Input: part model. Units: mm. Frame: model coordinates. A direction names the side the tool comes from. Give positions to 0.01 mm unless a question says otherwise; leave off trailing zeros. Order: outer loops, then holes, each group sorted by start corner. A loop starts at its lowest first (then second) coordinate and runs counter-clockwise, first axis right, second up. Notation, with made-up numbers: (0.5, 66.25) -> (38.5, 66.25) arc R35 cw to (38.5, 103.25) -> close; hole circle Ø6 at (89.25, 17). An arc over 180 degrees is marked (long way). Use a Markdown table: item, result. Add a question column.
from build123d import *

# Parameters (mm, degrees)
SKETCH1_W           = 115
SKETCH1_H           = 30
BOSS_EXTRUDE1_DEPTH = 10.5
CUT_EXTRUDE1_START  = 3
SKETCH2_R           = 11.1
CUT_EXTRUDE1_DEPTH  = 10.5
SKETCH3_R           = 6
CUT_EXTRUDE4_DEPTH  = 10.5
BOSS_EXTRUDE2_DEPTH = 10.5
SKETCH6_R           = 2.25
CUT_EXTRUDE5_DEPTH  = 10.5
SKETCH7_R           = 3
CUT_EXTRUDE6_DEPTH  = 7.5
CUT_EXTRUDE7_DEPTH  = 28.5
FILLET1_R           = 6
FILLET2_RADIUS      = 15
FILLET2_LENGTH      = 10.5


with BuildPart() as part:
    # Sketch1 → Boss-Extrude1 (new body)
    with BuildSketch(Plane(origin=(0, 0, 0), x_dir=(1, 0, 0), z_dir=(0, 1, 0))):
        Rectangle(SKETCH1_W, SKETCH1_H)
    extrude(amount=BOSS_EXTRUDE1_DEPTH)

    # Sketch2 → Cut-Extrude1 (cut)
    with BuildSketch(Plane(origin=(0, 0, 0), x_dir=(1, 0, 0), z_dir=(0, 1, 0)).offset(CUT_EXTRUDE1_START)):
        with Locations(Location((42.5, 0, 0), (0, 0, 90))):
            Circle(SKETCH2_R)
    extrude(amount=CUT_EXTRUDE1_DEPTH, mode=Mode.SUBTRACT)

    # Sketch3 → Cut-Extrude4 (cut)
    with BuildSketch(Plane(origin=(0, 0, 0), x_dir=(1, 0, 0), z_dir=(0, 1, 0))):
        with Locations(Location((42.5, 0, 0), (0, 0, 90))):
            Circle(SKETCH3_R)
    extrude(amount=CUT_EXTRUDE4_DEPTH, mode=Mode.SUBTRACT)

    # Sketch5 → Boss-Extrude2 (add)
    with BuildSketch(Plane(origin=(0, 0, 0), x_dir=(1, 0, 0), z_dir=(0, 1, 0))):
        Polygon((-57.5, 15), (-57.5, 25), (-37.5, 25), (-37.5, -25), (-57.5, -25), (-57.5, -15), align=None)
    extrude(amount=BOSS_EXTRUDE2_DEPTH)

    # Sketch6 → Cut-Extrude5 (cut)
    with BuildSketch(Plane(origin=(0, 10.5, 0), x_dir=(1, 0, 0), z_dir=(0, 1, 0))):
        with Locations(Location((-47.5, -15, 0), (0, 0, 270))):
            Circle(SKETCH6_R)
        with Locations(Location((-47.5, 15, 0), (0, 0, 270))):
            Circle(SKETCH6_R)
    extrude(amount=-CUT_EXTRUDE5_DEPTH, mode=Mode.SUBTRACT)

    # Sketch7 → Cut-Extrude6 (cut)
    with BuildSketch(Plane(origin=(0, 10.5, 0), x_dir=(1, 0, 0), z_dir=(0, 1, 0))):
        with Locations(Location((-47.5, 15, 0), (0, 0, 270))):
            Circle(SKETCH7_R)
        with Locations(Location((-47.5, -15, 0), (0, 0, 270))):
            Circle(SKETCH7_R)
    extrude(amount=-CUT_EXTRUDE6_DEPTH, mode=Mode.SUBTRACT)

    # Sketch8 → Cut-Extrude7 (cut)
    with BuildSketch(Plane(origin=(0, 10.5, 0), x_dir=(1, 0, 0), z_dir=(0, 1, 0))):
        Polygon((-37.5, 15), (-27.5, 7.5), (17.022877386, 7.5), (27.5, 15), align=None)
        Polygon((-37.5, -15), (27.5, -15), (17.022877386, -7.5), (-27.5, -7.5), align=None)
    extrude(amount=-CUT_EXTRUDE7_DEPTH, mode=Mode.SUBTRACT)

    # Fillet1
    fillet1_edges = [part.edges().sort_by_distance(p)[0] for p in [
        (-37.5, 5.25, -15),
        (-37.5, 5.25, 15),
        (-37.5, 5.25, 25),
        (-37.5, 5.25, -25),
        (27.5, 5.25, -15),
        (17.022877386, 5.25, -7.5),
        (-27.5, 5.25, -7.5),
        (-27.5, 5.25, 7.5),
        (17.022877386, 5.25, 7.5),
        (27.5, 5.25, 15),
    ]]
    fillet(fillet1_edges, radius=FILLET1_R)

    # Fillet2: full round fillet: the end face becomes a half cylinder, R = half its width
    fillet2_face = Plane((57.5, 5.25, 0), x_dir=(0, -1, 0), z_dir=(1, 0, 0))  # on the end face: x along it, z out of the body
    fillet2_slab = fillet2_face.offset(-FILLET2_RADIUS / 2) * Box(FILLET2_LENGTH, 2 * FILLET2_RADIUS, FILLET2_RADIUS, mode=Mode.PRIVATE)  # the body's end, R deep
    fillet2_round = Plane((42.5, 5.25, 0), x_dir=(1, 0, 0), z_dir=(0, -1, 0)) * Cylinder(FILLET2_RADIUS, FILLET2_LENGTH, mode=Mode.PRIVATE)  # its axis R under the face
    add(fillet2_slab - fillet2_round, mode=Mode.SUBTRACT)


solid = part.part
Q1. Ray query, line 1 (Z direction, x = 42.5, y = 1); line 2 (X direction, y = 6.25, z = 0); line 3 (Z direction, x = -26, y = 6.75). Return the intervals inside material, ascending.
Q2. Access query for faces 1 (the flat face through (36, 5, 15)), 2 (the cylindrical face through (31.494, 6.698, 1.445)), 3 (the flat face through (-5, 5, -7.5)), 4 (the flat face through (-5, 5, 7.5)). Directions: +Z, -Z, +X, -X, +Y, -Y. A direction counts if a zero-diameter tool reaches every point of the face in a straight line with its end or side. Return the directions, or none.
Q3. Section query A-A (z = 0). Return loops of the section in (x, y).
Q4. Draft query along Z for faces 5 (the flat face through (22.313, 5.324, 11.287)), 6 (the flat face through (22.21, 5.324, -11.213)), 7 (the cylindrical face through (48.357, 1.479, 1.301)). Return one class per face: +Z half, -Z half, draft (parallel to the pull), parting line (faces both ways), or undercut.
Q5. Section query C-C (x = 46). Return loops of the section in (y, z).
Q6. Section query B-B (y = 4.5). Return loops of the section in (x, z), plus the area to 3 significant figures.
Q7. Section query D-D (x = -22). Return loops of the section in (y, z), plus the area to 4 significant figures.
Q8. First-contact query: pin 1 (5 mm diameter, centred on x = -6, y = 6.5, fed in from -Z); pin 2 (3 mm diameter, centred on x = 31, y = 7.5, fed in from +Z); pin 3 (1.8 mm diameter, centred on x = -49, z = 16, fed in from +Y). Flat tips, straight axial feed; report the tip coordinate or a pass-through.
Solution:
| question | item | result |
|---|---|---|
| 1 | line 1 | z = -15 to -6, 6 to 15 |
| 1 | line 2 | x = -57.5 to 31.4, 53.6 to 57.5 |
| 1 | line 3 | z = -7.52 to 7.52 |
| 2 | face 1 | +Z, +X, +Y, -Y |
| 2 | face 2 | +Y |
| 2 | face 3 | -Z, +Y, -Y |
| 2 | face 4 | +Z, +Y, -Y |
| 3 | outline | (-57.5, 0) -> (36.5, 0) -> (36.5, 3) -> (31.4, 3) -> (31.4, 10.5) -> (-57.5, 10.5) -> close; (48.5, 0) -> (57.5, 0) -> (57.5, 10.5) -> (53.6, 10.5) -> (53.6, 3) -> (48.5, 3) -> close |
| 4 | face 5 | +Z half |
| 4 | face 6 | -Z half |
| 4 | face 7 | undercut |
| 5 | outline | (0, -14.59) -> (10.5, -14.59) -> (10.5, -10.53) -> (3, -10.53) -> (3, -4.87) -> (0, -4.87) -> close; (0, 4.87) -> (3, 4.87) -> (3, 10.53) -> (10.5, 10.53) -> (10.5, 14.59) -> (0, 14.59) -> close |
| 6 | outline | (-57.5, -25) -> (-43.5, -25) arc R6 ccw to (-37.5, -19) -> (-37.5, -18) arc R6 cw to (-35.1, -13.2) -> (-29.1, -8.7) arc R6 cw to (-25.5, -7.5) -> (15.1, -7.5) arc R6 cw to (18.59, -8.62) -> (25.93, -13.88) arc R6 ccw to (29.43, -15) -> (42.5, -15) arc R15 ccw to (42.5, 15) -> (29.43, 15) arc R6 ccw to (25.93, 13.88) -> (18.59, 8.62) arc R6 cw to (15.1, 7.5) -> (-25.5, 7.5) arc R6 cw to (-29.1, 8.7) -> (-35.1, 13.2) arc R6 cw to (-37.5, 18) -> (-37.5, 19) arc R6 ccw to (-43.5, 25) -> (-57.5, 25) -> close; hole circle Ø6 at (-47.5, -15); hole circle Ø6 at (-47.5, 15); hole circle Ø22.2 at (42.5, 0) |
| 6 | area | 2,480 mm² |
| 7 | outline | (0, -7.5) -> (10.5, -7.5) -> (10.5, 7.5) -> (0, 7.5) -> close |
| 7 | area | 157.5 mm² |
| 8 | pin 1 | stops at z = -7.5 |
| 8 | pin 2 | stops at z = 15 |
| 8 | pin 3 | stops at y = 3 |
